from build123d import *

# Parameters (mm, degrees)
BOSS_EXTRUDE1_DEPTH     = 150
FILLET1_R               = 48
CUT_EXTRUDE1_DEPTH      = 201
CUT_EXTRUDE1_DEPTH_BACK = 201
BOSS_EXTRUDE2_DEPTH     = 150
FILLET2_R               = 48
BOSS_EXTRUDE3_DEPTH     = 150
FILLET3_R               = 2
FILLET4_R               = 0.5


with BuildPart() as part:
    # Sketch1 → Boss-Extrude1 (new body)
    with BuildSketch(Plane(origin=(0, 0, 0), x_dir=(1, 0, 0), z_dir=(0, 1, 0))):
        Polygon((0, 0), (50, 86.602540378), (100, 0), align=None)
    extrude(amount=BOSS_EXTRUDE1_DEPTH)

    # Fillet1
    fillet1_edges = [part.edges().sort_by_distance(p)[0] for p in [
        (0, 75, 0),
    ]]
    fillet(fillet1_edges, radius=FILLET1_R)

    # Sketch3 → Cut-Extrude1 (cut, two sides: drawn at the far end of the back side and taken through both)
    with BuildSketch(Plane.XZ.offset(-CUT_EXTRUDE1_DEPTH_BACK)):
        with BuildLine():
            Line((45.899346401, -69.5), (52.886751346, -81.602540378))
            Line((52.886751346, -81.602540378), (97.113248654, -5))
            Line((97.113248654, -5), (83.138438763, -5))
            ThreePointArc((83.138438763, -5), (45.899346401, -26.5), (45.899346401, -69.5))
        make_face()
    extrude(amount=CUT_EXTRUDE1_DEPTH + CUT_EXTRUDE1_DEPTH_BACK, mode=Mode.SUBTRACT)

    # Sketch4 → Boss-Extrude2 (add)
    with BuildSketch(Plane(origin=(0, 0, 0), x_dir=(1, 0, 0), z_dir=(0, 1, 0))):
        Polygon((50, 86.602540378), (57.886751346, 90.262794416), (52.886751346, 81.602540378), align=None)
        Polygon((97.113248654, 5), (100, 0), (107.113248654, 5), align=None)
    extrude(amount=BOSS_EXTRUDE2_DEPTH)

    # Fillet2
    # the kernel refuses this fillet: 48 mm, written as the material it takes off along each edge
    with BuildSketch(Plane(origin=(50, -35.543700884, -86.602540378), x_dir=(-0.5000000000000046, 0, 0.8660254037844362), z_dir=(0, 1, 0))) as fillet2_piece_1:
        with BuildLine():
            CenterArc((14.217480354, 48), FILLET2_R, 243.615670251, 26.384329749)
            Line((-7.113248654, 5), (-7.539863234, 4.14))
            ThreePointArc((-7.539863234, 4.14), (-4.108682958, 1.714613937), (-0.552058631, -0.785386063))
            Line((-0.552058631, -0.785386063), (0, -0.96))
            Line((0, -0.96), (14.217480354, -0.96))
            Line((14.217480354, -0.96), (14.217480354, 0))
        make_face()
    extrude(amount=221.087401768, mode=Mode.SUBTRACT)
    with BuildSketch(Plane(origin=(100, -35.543700884, 0), x_dir=(-1, 0, 0), z_dir=(0, 1, 0))) as fillet2_piece_2:
        with BuildLine():
            CenterArc((14.217480354, -48), FILLET2_R, 90, 26.384329749)
            Line((-7.113248654, -5), (-7.539863234, -4.14))
            ThreePointArc((-7.539863234, -4.14), (-4.108682958, -1.714613937), (-0.552058631, 0.785386063))
            Line((-0.552058631, 0.785386063), (0, 0.96))
            Line((0, 0.96), (14.217480354, 0.96))
            Line((14.217480354, 0.96), (14.217480354, 0))
        make_face()
    extrude(amount=221.087401768, mode=Mode.SUBTRACT)

    # Sketch5 → Boss-Extrude3 (add)
    with BuildSketch(Plane(origin=(0, 0, 0), x_dir=(1, 0, 0), z_dir=(0, 1, 0))):
        Polygon((54.717765705, 36.671999128), (57.142636836, 36.339948321), (57.642636836, 35.473922917), (43.850262737, 27.510892018), (43.385383074, 28.397194158), (54.717765705, 34.939948321), align=None)
        Polygon((59.542636836, 32.183026382), (60.042636836, 31.317000979), (58.944560624, 28.950975575), (57.444560624, 29.817000979), (45.904890393, 23.154569264), (45.509810975, 24.081170595), align=None)
    extrude(amount=BOSS_EXTRUDE3_DEPTH)

    # Fillet3
    fillet3_edges = [part.edges().sort_by_distance(p)[0] for p in [
        (44.534132149, 75, -29.060424746),
        (47.434132149, 75, -24.037477404),
    ]]
    fillet(fillet3_edges, radius=FILLET3_R)

    # Fillet4
    fillet4_edges = [part.edges().sort_by_distance(p)[0] for p in [
        (54.717765705, 75, -36.671999128),
        (58.944560624, 75, -28.950975575),
    ]]
    fillet(fillet4_edges, radius=FILLET4_R)


solid = part.part
Can you work these out from the model? Positions are in its coordinate system, mm. A direction names the side the tool comes from. Coordinates: 2 decimals unless noted, no trailing zeros. Order: outer loops, then holes, each group sorted by start corner. A loop starts at its lowest first (then second) coordinate and runs counter-clockwise, first axis right, second up. Notation, with made-up numbers: M -32,-32.75 L -11,-32.75 A18 ccw -11,-3.75 Z; hole C 0,88 d9. An arc over 180 degrees is marked long. Answer as CSV lines item,"result".
(1) On a 3-axis mill with a long thin cutter (end or side, diameter ignored), from which of +Z, -Z, +X, -X, +Y, -Y can I reach the whole of each face in a straight line? I mean faces 1 (the flat face through (53.13, 73.95, -28.48)), 2 (the flat face through (55, 150, -35)), 3 (the cylindrical face through (64.156, 76.05, -9.417)), 4 (the cylindrical face through (41.222, 76.05, -24.612)), 5 (the flat face through (95, 76, -5)). Say none if no direction works.
Geometry check:
face 1,"+Y, -Y"
face 2,"+Z, -Z, +X, -X, +Y"
face 3,"+X, +Y, -Y"
face 4,"-X, +Y, -Y"
face 5,"-Z, +X, +Y, -Y"
(2) I'm going to push flat-ended pins straight in: pin 1 (10 mm diameter, centred on x = 52, y = 42.5, fed in from -Z); pin 2 (1 mm diameter, centred on x = 56, y = 93, fed in from -Z); pin 3 (12 mm diameter, centred on y = 17, z = -48.5, fed in from +X). Where does each tip first touch, or does it pass through?
Geometry check:
pin 1,"z = -89.66"
pin 2,"z = -89.31"
pin 3,"x = 40.63"
(3) Suppose I cut it at C-C on x = 95.5. Please give me the cut outline in (y, z), plus the area to 3 significant figures.
Geometry check:
outline,"M 0,-5 L 150,-5 L 150,-0.99 L 0,-0.99 Z"
area,"601 mm^2"
(4) Suppose I cut it at A-A on y = 47. Please give me the cut outline in (x, z).
Geometry check:
outline,"M 41.57,-72 L 42.89,-74.29 A48 ccw 57.89,-90.26 L 45.9,-69.5 A43 cw 43.6,-31.1 A2 cw 46.44,-30.16 L 54.72,-34.94 L 54.72,-36.1 A0.5 ccw 55.29,-36.59 L 57.14,-36.34 L 57.64,-35.47 L 44.99,-28.17 A43 cw 46.89,-24.88 L 59.54,-32.18 L 60.04,-31.32 L 59.17,-29.45 A0.5 ccw 58.47,-29.22 L 57.44,-29.82 L 49.34,-25.14 A2 cw 48.74,-22.2 A43 cw 83.14,-5 L 107.11,-5 A48 ccw 85.78,0 L 83.14,0 A48 ccw Z"
(5) Please list where these lines run through material, in increasing order: L1, parallel to Z at x = 47, y = 37; L2, parallel to Z at x = 49, y = 51; L3, parallel to Z at x = 54.5, y = 12.
Geometry check:
L1,"-80.3 to -71.41, -30.48 to -29.33, -24.94 to -16.41"
L2,"-82.64 to -74.87, -31.64 to -30.48, -26.1 to -24.89, -21.85 to -14.26"
L3,"-87.79 to -84.4, -34.81 to -33.66, -29.27 to -28.12, -15.92 to -9.48"
(6) If we mould it in two halves opening along Z, with no side actions, what happens to faces 6 (the cylindrical face through (96.586, 73.95, -1.232)), 7 (the flat face through (51.4, 73.95, -31.87)), 8 (the flat face through (55, 0, -35))? For each: released by +Z, released by -Z, zero draft, split by the parting line, or undercut.
Geometry check:
face 6,"released by +Z"
face 7,"undercut"
face 8,"zero draft"
(7) Suppose I cut it at B-B on z = -55. Please give me the cut outline in (x, y), plus the area to 3 significant figures.
Geometry check:
outline,"M 35.65,0 L 40.71,0 L 40.71,150 L 35.65,150 Z"
area,"759 mm^2"
